```python
from build123d import *

# Parameters (mm, degrees)
SKETCH1_W           = 25.4
SKETCH1_H           = 25.4
BOSS_EXTRUDE1_DEPTH = 3.81
FILLET1_R           = 2.1082
SKETCH4_W           = 6.35
SKETCH4_H           = 2.54
SKETCH4_W_2         = 2.54
SKETCH4_H_2         = 6.35
BOSS_EXTRUDE2_DEPTH = 2.54


with BuildPart() as part:
    # Sketch1 → Boss-Extrude1 (new body, symmetric)
    with BuildSketch(Plane.XY):
        Rectangle(SKETCH1_W, SKETCH1_H)
    extrude(amount=BOSS_EXTRUDE1_DEPTH, both=True)

    # Sketch3 → CSK for 1/4 Flat Head Socket Cap Screw1 (revolve, cut)
    with BuildSketch(Plane(origin=(0, 0, 3.81), x_dir=(0, -1, 0), z_dir=(1, 0, 0))):
        Polygon((0, 0), (0, 7.62), (3.2639, 7.62), (3.2639, 5.019052874), (7.6268961, 0), align=None)
    revolve(axis=Axis((0, 0, 10.16), (0, 0, -1)), mode=Mode.SUBTRACT)

    # Fillet1
    fillet1_edges = [part.edges().sort_by_distance(p)[0] for p in [
        (-12.7, 0, 3.81),
        (0, -12.7, 3.81),
        (12.7, 0, 3.81),
        (12.7, -12.7, 0),
        (-12.7, -12.7, 0),
        (-12.7, 12.7, 0),
        (12.7, 12.7, 0),
        (0, 12.7, 3.81),
    ]]
    fillet(fillet1_edges, radius=FILLET1_R)

    # Sketch4 → Boss-Extrude2 (add)
    with BuildSketch(Plane(origin=(0, 0, -3.81), x_dir=(-1, 0, 0), z_dir=(0, 0, -1))):
        with Locations((0, 11.43)):
            Rectangle(SKETCH4_W, SKETCH4_H)
        with Locations((-11.43, 0)):
            Rectangle(SKETCH4_W_2, SKETCH4_H_2)
        with Locations((11.43, 0)):
            Rectangle(SKETCH4_W_2, SKETCH4_H_2)
        with Locations((0, -11.43)):
            Rectangle(SKETCH4_W, SKETCH4_H)
    extrude(amount=BOSS_EXTRUDE2_DEPTH)


solid = part.part
```
Can you work these out from the model? Positions are in its coordinate system, mm. A direction names the side the tool comes from. Coordinates: 2 decimals unless noted, no trailing zeros. Loops run counter-clockwise (first coordinate to the right, second up) from the corner with the lowest first, then second, coordinate; pieces in that order, holes last.
1) Thinking about a two-plate mould opening in Y: for faces 1 (the flat face through (-11, -3.175, -5)), 2 (the cylindrical face through (0.148, 12.099, 3.176)), 3 (the cylindrical face through (3.186, 0.708, -2.491)), which applies, pulls with the +Y half, pulls with the -Y half, needs draft (parallel to the pull), parting line crosses it, or undercut?
2) Imagine slicing it at C-C on z = 1. List the corners of the cut face in (x, y) for me, plus the area to 3 significant figures.
3) For pin 1 (1 mm diameter, centred on x = -4.5, y = 3, fed in from +Z); pin 2 (1.3 mm diameter, centred on x = -11, z = -5.5, fed in from -Y) (3 decimals); pin 3 (2 mm diameter, centred on y = 11.5, z = -5.5, fed in from +X) (3 decimals), each with a flat end and sliding along its axis, tell me the tip position at first contact or that it passes through.
4) I need wall thicknesses on probe 1 along Y at (x, z) = (1, -5.75); probe 2 along X at (y, z) = (0, -2.85). Which ranges of each line are inside material? Lowest first, please.
5) Imagine slicing it at D-D on x = -9.5. List the corners of the cut face in (y, z) for me.
6) Which directions (+Z, -Z, +X, -X, +Y, -Y) give clear straight access to the entire face, cutting with the end or side of a thin tool? Please do faces 4 (the flat face through (11, -3.175, -5)), 5 (the flat face through (-3.175, 11, -5)), 6 (the flat face through (-11, 3.175, -5)), 7 (the flat face through (3.175, -11, -5)).
7) Imagine slicing it at A-A on x = 0. List the corners of the cut face in (y, z) for me, plus the area to 3 significant figures.
Completed:
1. face 1: pulls with the -Y half
1. face 2: pulls with the +Y half
1. face 3: undercut
2. outline: (-12.7, -10.59) arc R2.11 ccw to (-10.59, -12.7) - (10.59, -12.7) arc R2.11 ccw to (12.7, -10.59) - (12.7, 10.59) arc R2.11 ccw to (10.59, 12.7) - (-10.59, 12.7) arc R2.11 ccw to (-12.7, 10.59) - close; hole circle Ø10.37 at (0, 0)
2. area: 557 mm2
3. pin 1: stops at z = 1.83
3. pin 2: stops at y = -3.175
3. pin 3: stops at x = 3.175
4. probe 1: y = -12.7 to -10.16, 10.16 to 12.7
4. probe 2: x = -12.7 to -3.26, 3.26 to 12.7
5. outline: (-12.7, -3.81) - (12.7, -3.81) - (12.7, 1.7) arc R2.11 ccw to (10.59, 3.81) - (-10.59, 3.81) arc R2.11 ccw to (-12.7, 1.7) - close
6. face 4: -Z, +X, -X, -Y
6. face 5: -Z, -X, +Y, -Y
6. face 6: -Z, +X, -X, +Y
6. face 7: -Z, +X, +Y, -Y
7. outline: (-12.7, -6.35) - (-10.16, -6.35) - (-10.16, -3.81) - (-3.26, -3.81) - (-3.26, -1.21) - (-7.63, 3.81) - (-10.59, 3.81) arc R2.11 ccw to (-12.7, 1.7) - close; (3.26, -3.81) - (10.16, -3.81) - (10.16, -6.35) - (12.7, -6.35) - (12.7, 1.7) arc R2.11 ccw to (10.59, 3.81) - (7.63, 3.81) - (3.26, -1.21) - close
7. area: 133 mm2
